from build123d import *

# Parameters (mm, degrees)
CYLINDER1945_R               = 1.5
CYLINDER1945_DEPTH           = 20
CYLINDER1945_PLACEMENT_ANGLE = 67.5
CYLINDER1943_R               = 1.5
CYLINDER1943_DEPTH           = 20
CYLINDER1943_PLACEMENT_ANGLE = 112.5
CYLINDER1936_R               = 1.5
CYLINDER1936_DEPTH           = 20
CYLINDER1936_PLACEMENT_ANGLE = 157.5
CYLINDER1952_R               = 1.5
CYLINDER1952_DEPTH           = 20
CYLINDER1952_PLACEMENT_ANGLE = 202.5
CYLINDER1946_R               = 1.5
CYLINDER1946_DEPTH           = 20
CYLINDER1946_PLACEMENT_ANGLE = -112.5
CYLINDER1938_R               = 1.5
CYLINDER1938_DEPTH           = 20
CYLINDER1938_PLACEMENT_ANGLE = 67.5
CYLINDER1935_R               = 1.5
CYLINDER1935_DEPTH           = 20
CYLINDER1935_PLACEMENT_ANGLE = 22.5
CYLINDER1941_R               = 1.5
CYLINDER1941_DEPTH           = 20
CYLINDER1941_PLACEMENT_ANGLE = 22.5
BOX442_W                     = 6
BOX442_H                     = 6
BOX442_DEPTH                 = 2
BOX442_PLACEMENT_ANGLE       = 67.5
BOX437_W                     = 6
BOX437_H                     = 6
BOX437_DEPTH                 = 2
BOX437_PLACEMENT_ANGLE       = 112.5
BOX447_W                     = 6
BOX447_H                     = 6
BOX447_DEPTH                 = 2
BOX447_PLACEMENT_ANGLE       = 157.5
BOX445_W                     = 6
BOX445_H                     = 6
BOX445_DEPTH                 = 2
BOX445_PLACEMENT_ANGLE       = 202.5
BOX446_W                     = 6
BOX446_H                     = 6
BOX446_DEPTH                 = 2
BOX446_PLACEMENT_ANGLE       = -112.5
BOX449_W                     = 6
BOX449_H                     = 6
BOX449_DEPTH                 = 2
BOX449_PLACEMENT_ANGLE       = 67.5
BOX440_W                     = 6
BOX440_H                     = 6
BOX440_DEPTH                 = 2
BOX440_PLACEMENT_ANGLE       = 22.5
BOX443_W                     = 6
BOX443_H                     = 6
BOX443_DEPTH                 = 2
BOX443_PLACEMENT_ANGLE       = 22.5
TUBE085_R                    = 32
TUBE085_R_2                  = 26
TUBE085_DEPTH                = 6


with BuildPart() as obj1:
    # Cylinder1945 → Cylinder1945 (new body)
    with BuildSketch(Plane.XY):
        Circle(CYLINDER1945_R)
    extrude(amount=CYLINDER1945_DEPTH)


with BuildPart() as obj1_1:
    # Cylinder1945 placement: moved
    add(obj1.part.moved(Location((11.09782, 26.792506, -10))).rotate(Axis((11.09782, 26.792506, -10), (0, 0, 1)), CYLINDER1945_PLACEMENT_ANGLE))


with BuildPart() as obj2:
    # Cylinder1943 → Cylinder1943 (new body)
    with BuildSketch(Plane.XY):
        Circle(CYLINDER1943_R)
    extrude(amount=CYLINDER1943_DEPTH)


with BuildPart() as obj2_1:
    # Cylinder1943 placement: moved
    add(obj2.part.moved(Location((-11.09782, 26.792506, -10))).rotate(Axis((-11.09782, 26.792506, -10), (0, 0, 1)), CYLINDER1943_PLACEMENT_ANGLE))


with BuildPart() as obj3:
    # Cylinder1936 → Cylinder1936 (new body)
    with BuildSketch(Plane.XY):
        Circle(CYLINDER1936_R)
    extrude(amount=CYLINDER1936_DEPTH)


with BuildPart() as obj3_1:
    # Cylinder1936 placement: moved
    add(obj3.part.moved(Location((-26.792506, 11.09782, -10))).rotate(Axis((-26.792506, 11.09782, -10), (0, 0, 1)), CYLINDER1936_PLACEMENT_ANGLE))


with BuildPart() as obj4:
    # Cylinder1952 → Cylinder1952 (new body)
    with BuildSketch(Plane.XY):
        Circle(CYLINDER1952_R)
    extrude(amount=CYLINDER1952_DEPTH)


with BuildPart() as obj4_1:
    # Cylinder1952 placement: moved
    add(obj4.part.moved(Location((-26.792506, -11.09782, -10))).rotate(Axis((-26.792506, -11.09782, -10), (0, 0, 1)), CYLINDER1952_PLACEMENT_ANGLE))


with BuildPart() as obj5:
    # Cylinder1946 → Cylinder1946 (new body)
    with BuildSketch(Plane.XY):
        Circle(CYLINDER1946_R)
    extrude(amount=CYLINDER1946_DEPTH)


with BuildPart() as obj5_1:
    # Cylinder1946 placement: moved
    add(obj5.part.moved(Location((-11.09782, -26.792506, -10))).rotate(Axis((-11.09782, -26.792506, -10), (0, 0, 1)), CYLINDER1946_PLACEMENT_ANGLE))


with BuildPart() as obj6:
    # Cylinder1938 → Cylinder1938 (new body)
    with BuildSketch(Plane.XY):
        Circle(CYLINDER1938_R)
    extrude(amount=CYLINDER1938_DEPTH)


with BuildPart() as obj6_1:
    # Cylinder1938 placement: moved
    add(obj6.part.moved(Location((11.09782, -26.792506, -10))).rotate(Axis((11.09782, -26.792506, -10), (0, 0, -1)), CYLINDER1938_PLACEMENT_ANGLE))


with BuildPart() as obj7:
    # Cylinder1935 → Cylinder1935 (new body)
    with BuildSketch(Plane.XY):
        Circle(CYLINDER1935_R)
    extrude(amount=CYLINDER1935_DEPTH)


with BuildPart() as obj7_1:
    # Cylinder1935 placement: moved
    add(obj7.part.moved(Location((26.792506, -11.09782, -10))).rotate(Axis((26.792506, -11.09782, -10), (0, 0, -1)), CYLINDER1935_PLACEMENT_ANGLE))


with BuildPart() as compound883:
    # Cylinder1941 → Cylinder1941 (new body)
    with BuildSketch(Plane.XY):
        Circle(CYLINDER1941_R)
    extrude(amount=CYLINDER1941_DEPTH)


with BuildPart() as compound883_1:
    # Cylinder1941 placement: moved
    add(compound883.part.moved(Location((26.792506, 11.09782, -10))).rotate(Axis((26.792506, 11.09782, -10), (0, 0, 1)), CYLINDER1941_PLACEMENT_ANGLE))

    # Compound883: union obj1, obj2, obj3, obj4, obj5, obj6, obj7
    add(obj1_1.part)
    add(obj2_1.part)
    add(obj3_1.part)
    add(obj4_1.part)
    add(obj5_1.part)
    add(obj6_1.part)
    add(obj7_1.part)


with BuildPart() as krychle442:
    # Box442 → Box442 (new body)
    with BuildSketch(Plane.XY):
        with Locations((3, 3)):
            Rectangle(BOX442_W, BOX442_H)
    extrude(amount=BOX442_DEPTH)


with BuildPart() as krychle442_1:
    # Box442 placement: moved
    add(krychle442.part.moved(Location((12.721408, 22.872818, -2))).rotate(Axis((12.721408, 22.872818, -2), (0, 0, 1)), BOX442_PLACEMENT_ANGLE))


with BuildPart() as krychle437:
    # Box437 → Box437 (new body)
    with BuildSketch(Plane.XY):
        with Locations((3, 3)):
            Rectangle(BOX437_W, BOX437_H)
    extrude(amount=BOX437_DEPTH)


with BuildPart() as krychle437_1:
    # Box437 placement: moved
    add(krychle437.part.moved(Location((-7.178131, 25.168918, -2))).rotate(Axis((-7.178131, 25.168918, -2), (0, 0, 1)), BOX437_PLACEMENT_ANGLE))


with BuildPart() as krychle447:
    # Box447 → Box447 (new body)
    with BuildSketch(Plane.XY):
        with Locations((3, 3)):
            Rectangle(BOX447_W, BOX447_H)
    extrude(amount=BOX447_DEPTH)


with BuildPart() as krychle447_1:
    # Box447 placement: moved
    add(krychle447.part.moved(Location((-22.872818, 12.721408, -2))).rotate(Axis((-22.872818, 12.721408, -2), (0, 0, 1)), BOX447_PLACEMENT_ANGLE))


with BuildPart() as krychle445:
    # Box445 → Box445 (new body)
    with BuildSketch(Plane.XY):
        with Locations((3, 3)):
            Rectangle(BOX445_W, BOX445_H)
    extrude(amount=BOX445_DEPTH)


with BuildPart() as krychle445_1:
    # Box445 placement: moved
    add(krychle445.part.moved(Location((-25.168918, -7.178131, -2))).rotate(Axis((-25.168918, -7.178131, -2), (0, 0, 1)), BOX445_PLACEMENT_ANGLE))


with BuildPart() as krychle446:
    # Box446 → Box446 (new body)
    with BuildSketch(Plane.XY):
        with Locations((3, 3)):
            Rectangle(BOX446_W, BOX446_H)
    extrude(amount=BOX446_DEPTH)


with BuildPart() as krychle446_1:
    # Box446 placement: moved
    add(krychle446.part.moved(Location((-12.721408, -22.872818, -2))).rotate(Axis((-12.721408, -22.872818, -2), (0, 0, 1)), BOX446_PLACEMENT_ANGLE))


with BuildPart() as krychle449:
    # Box449 → Box449 (new body)
    with BuildSketch(Plane.XY):
        with Locations((3, 3)):
            Rectangle(BOX449_W, BOX449_H)
    extrude(amount=BOX449_DEPTH)


with BuildPart() as krychle449_1:
    # Box449 placement: moved
    add(krychle449.part.moved(Location((7.178131, -25.168918, -2))).rotate(Axis((7.178131, -25.168918, -2), (0, 0, -1)), BOX449_PLACEMENT_ANGLE))


with BuildPart() as krychle440:
    # Box440 → Box440 (new body)
    with BuildSketch(Plane.XY):
        with Locations((3, 3)):
            Rectangle(BOX440_W, BOX440_H)
    extrude(amount=BOX440_DEPTH)


with BuildPart() as krychle440_1:
    # Box440 placement: moved
    add(krychle440.part.moved(Location((22.872818, -12.721408, -2))).rotate(Axis((22.872818, -12.721408, -2), (0, 0, -1)), BOX440_PLACEMENT_ANGLE))


with BuildPart() as compound876:
    # Box443 → Box443 (new body)
    with BuildSketch(Plane.XY):
        with Locations((3, 3)):
            Rectangle(BOX443_W, BOX443_H)
    extrude(amount=BOX443_DEPTH)


with BuildPart() as compound876_1:
    # Box443 placement: moved
    add(compound876.part.moved(Location((25.168918, 7.178131, -2))).rotate(Axis((25.168918, 7.178131, -2), (0, 0, 1)), BOX443_PLACEMENT_ANGLE))

    # Compound876: union Krychle442, Krychle437, Krychle447, Krychle445, Krychle446, Krychle449, Krychle440
    add(krychle442_1.part)
    add(krychle437_1.part)
    add(krychle447_1.part)
    add(krychle445_1.part)
    add(krychle446_1.part)
    add(krychle449_1.part)
    add(krychle440_1.part)


with BuildPart() as cut519:
    # Tube085 → Tube085 (new body)
    with BuildSketch(Plane.XY.offset(-6)):
        Circle(TUBE085_R)
        Circle(TUBE085_R_2, mode=Mode.SUBTRACT)
    extrude(amount=TUBE085_DEPTH)

    # Cut523: cut Compound876
    add(compound876_1.part, mode=Mode.SUBTRACT)

    # Cut519: cut Compound883
    add(compound883_1.part, mode=Mode.SUBTRACT)


solid = cut519.part
Check sheet for the modelled part. Datum: model origin and axes. Units: mm. A direction names the side the tool comes from. Round coordinates to 2 decimals unless told otherwise and drop trailing zeros. Loops run counter-clockwise (first coordinate to the right, second up) from the corner with the lowest first, then second, coordinate; pieces in that order, holes last.
1. Sectioned sample at A-A on y = 0. Record the boundary of the cut face in (x, z), and give its area (3 significant figures).
2. Mould release check, pull along X, two halves, no side actions. Record for faces 1 (the flat face through (27.838, -8.284, -1.014)), 2 (the flat face through (25.541, -13.827, -1.014)), 3 (the flat face through (-27.838, 8.284, -1.014)), 4 (the flat face through (-25.541, 13.827, -1.014)): released by +X, released by -X, zero draft, split by the parting line, or undercut.
3. Scan lines: probe 1 along Y at (x, z) = (-28, -3.6); probe 2 along X at (y, z) = (-27, -2.3); probe 3 along X at (y, z) = (10, -3.75). Record each from-to range of solid material in increasing order.
4. Sectioned sample at C-C on z = -2.85. Give the number of separate pieces and of enclosed holes in the cut face, and give its area (3 significant figures).
5. Set-up check for faces 5 (the flat face through (8.284, -27.838, -1.014)), 6 (the flat face through (13.827, -25.541, -1.014)), 7 (the flat face through (-25.541, -13.827, -1.014)): record each of +Z, -Z, +X, -X, +Y, -Y from which the full face is reachable in a straight line by a thin tool's end or side.
6. Gauge pin test, flat ends, axial feed: pin 1 Ø2.5 at (x, y) = (26.79, -11.1) entering from +Z; pin 2 Ø1.5 at (x, z) = (-22, -5) entering from +Y; pin 3 Ø1 at (y, z) = (-7, -3.5) entering from +X; pin 4 Ø4 at (x, y) = (-27, -10.5) entering from +Z. Record the tip position at first contact, or that the pin passes through.
Recorded:
1. outline: (-32, -6) - (-26, -6) - (-26, 0) - (-32, 0) - close; (26, -6) - (32, -6) - (32, 0) - (26, 0) - close
1. area: 72.0 mm2
2. face 1: undercut
2. face 2: released by +X
2. face 3: undercut
2. face 4: released by -X
3. probe 1: y = -15.49 to -11.99, -10.21 to 10.21, 11.99 to 15.49
3. probe 2: x = -17.18 to -12.58, -9.61 to 9.61, 12.58 to 17.18
3. probe 3: x = -30.4 to -27.81, -25.77 to -24, 24 to 25.77, 27.81 to 30.4
4. separate pieces: 1
4. enclosed holes: 9
4. area: 1,040 mm2
5. face 5: +Z
5. face 6: +Z, -Y
5. face 7: +Z, -X
6. pin 1: passes through
6. pin 2: stops at y = 23.93
6. pin 3: stops at x = 31.33
6. pin 4: stops at z = -2
